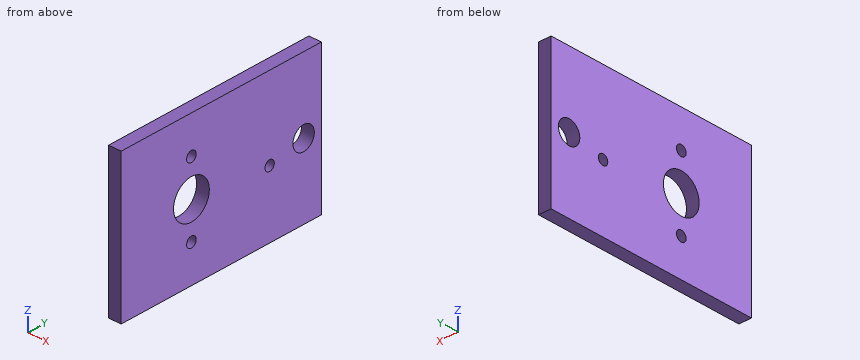
```python
from build123d import *

# Parameters (mm, degrees)
SKETCH1_W           = 50.8
SKETCH1_H           = 75
BOSS_EXTRUDE1_DEPTH = 4.4
SKETCH2_R           = 4
SKETCH2_R_2         = 6.7
SKETCH2_R_3         = 1.8
CUT_EXTRUDE1_DEPTH  = 46.505713927
SKETCH4_R           = 1.75
CUT_EXTRUDE2_DEPTH  = 46.505713927


with BuildPart() as part:
    # Sketch1 → Boss-Extrude1 (new body)
    with BuildSketch(Plane(origin=(0, 0, 0), x_dir=(0, 0, -1), z_dir=(1, 0, 0))):
        Rectangle(SKETCH1_W, SKETCH1_H)
    extrude(amount=BOSS_EXTRUDE1_DEPTH)

    # Sketch2 → Cut-Extrude1 (cut, through all)
    with BuildSketch(Plane(origin=(4.4, 0, 0), x_dir=(0, 0, -1), z_dir=(1, 0, 0))):
        with Locations((0, 30.794503628)):
            Circle(SKETCH2_R)
        with Locations((0, -11.205496372)):
            Circle(SKETCH2_R_2)
        with Locations((-12.565, -11.205496372)):
            Circle(SKETCH2_R_3)
        with Locations((12.565, -11.205496372)):
            Circle(SKETCH2_R_3)
    extrude(amount=-CUT_EXTRUDE1_DEPTH, mode=Mode.SUBTRACT)

    # Sketch4 → Cut-Extrude2 (cut, through all)
    with BuildSketch(Plane(origin=(4.4, 0, 0), x_dir=(0, 0, -1), z_dir=(1, 0, 0))):
        with Locations((2.63504704, 18.069503628)):
            Circle(SKETCH4_R)
    extrude(amount=-CUT_EXTRUDE2_DEPTH, mode=Mode.SUBTRACT)


solid = part.part
```
Input: part model. Units: mm. Frame: model coordinates. Give positions to 0.01 mm unless a question says otherwise; leave off trailing zeros. Order: outer loops, then holes, each group sorted by start corner. A loop starts at its lowest first (then second) coordinate and runs counter-clockwise, first axis right, second up.
1. Cut plane A-A (z = 0). Return loops of the section in (x, y).
Computed:
outline: (0, -37.5) - (4.4, -37.5) - (4.4, -17.91) - (0, -17.91) - close; (0, -4.51) - (4.4, -4.51) - (4.4, 26.79) - (0, 26.79) - close; (0, 34.79) - (4.4, 34.79) - (4.4, 37.5) - (0, 37.5) - close
2. Pin query (flat end, axial travel): pin 1 Ø2 at (y, z) = (18.07, -2.64) entering from -X. Return the tip coordinate at first contact, or that it passes through.
Computed:
pin 1: passes through
3. Line query: probe 1 along Y at (x, z) = (1.5, 0); probe 2 along Y at (x, z) = (1.25, 1); probe 3 along Y at (x, z) = (3.65, -1.5). Output: solid intervals per line, ascending.
Computed:
probe 1: y = -37.5 to -17.91, -4.51 to 26.79, 34.79 to 37.5
probe 2: y = -37.5 to -17.83, -4.58 to 26.92, 34.67 to 37.5
probe 3: y = -37.5 to -17.74, -4.68 to 16.74, 19.4 to 27.09, 34.5 to 37.5
4. Cut plane C-C (x = 2.75). State how many separate pieces and enclosed holes the cut face has, and give its area (3 significant figures).
Computed:
separate pieces: 1
enclosed holes: 5
area: 3,590 mm2
5. Cut plane B-B (y = -7). Return loops of the section in (x, z), and give its area (3 significant figures).
Computed:
outline: (0, -25.4) - (4.4, -25.4) - (4.4, -5.22) - (0, -5.22) - close; (0, 5.22) - (4.4, 5.22) - (4.4, 25.4) - (0, 25.4) - close
area: 178 mm2
